Check sheet for the modelled part. Datum: model origin and axes. Units: mm. A direction names the side the tool comes from. Coordinates: 2 decimals unless noted, no trailing zeros. Loops run counter-clockwise (first coordinate to the right, second up) from the corner with the lowest first, then second, coordinate; pieces in that order, holes last. Notation, with made-up numbers: M -25.75,65 L -19.75,65 A22 ccw -19.75,88 Z; hole C -27,72 d3. An arc over 180 degrees is marked long. Answer as CSV lines item,"result". Start each with the question number.
from build123d import *

# Parameters (mm, degrees)
BOSS_EXTRUDE1_DEPTH = 5
BOSS_EXTRUDE2_DEPTH = 3
SKETCH3_W           = 7.507408842
SKETCH3_H           = 20
BOSS_EXTRUDE3_DEPTH = 12
SKETCH5_W           = 19.5
SKETCH5_H           = 2.15
CUT_EXTRUDE2_DEPTH  = 18
CUT_EXTRUDE3_DEPTH  = 50.600358979


with BuildPart() as part:
    # Sketch1 → Boss-Extrude1 (new body)
    with BuildSketch(Plane(origin=(0, 0, 0), x_dir=(1, 0, 0), z_dir=(0, 1, 0))):
        Polygon((10.024698463, 8.496116817), (-10.024698463, 8.496116817), (-29.349158436, -10.828343156), (-17.64879837, -38.142135624), (17.64879837, -38.142135624), (29.349158436, -10.828343156), align=None)
        Polygon((9.196271338, 6.496116817), (-9.196271338, 6.496116817), (-26.977652736, -11.28526458), (-16.329759674, -36.142135624), (16.329759674, -36.142135624), (26.977652736, -11.28526458), align=None, mode=Mode.SUBTRACT)
    extrude(amount=BOSS_EXTRUDE1_DEPTH)

    # Sketch2 → Boss-Extrude2 (add)
    with BuildSketch(Plane(origin=(0, 0, 0), x_dir=(-1, 0, 0), z_dir=(0, -1, 0))):
        Polygon((17.64879837, -38.142135624), (-17.64879837, -38.142135624), (-29.349158436, -10.828343156), (-10.024698463, 8.496116817), (10.024698463, 8.496116817), (29.349158436, -10.828343156), align=None)
    extrude(amount=BOSS_EXTRUDE2_DEPTH)

    # Sketch3 → Boss-Extrude3 (add)
    with BuildSketch(Plane(origin=(0, -3, 0), x_dir=(-1, 0, 0), z_dir=(0, -1, 0))):
        with Locations((9.003704421, -17.503883183)):
            Rectangle(SKETCH3_W, SKETCH3_H)
        with Locations((-9.003704421, -17.503883183)):
            Rectangle(SKETCH3_W, SKETCH3_H)
    extrude(amount=BOSS_EXTRUDE3_DEPTH)

    # Sketch5 → Cut-Extrude2 (cut)
    with BuildSketch(Plane(origin=(0, 0, 7.503883183), x_dir=(-1, 0, 0), z_dir=(0, 0, -1))):
        with Locations((0, -11.925)):
            Rectangle(SKETCH5_W, SKETCH5_H)
    extrude(amount=-CUT_EXTRUDE2_DEPTH, mode=Mode.SUBTRACT)

    # Sketch6 → Cut-Extrude3 (cut, through all)
    with BuildSketch(Plane(origin=(0, -3, 0), x_dir=(-1, 0, 0), z_dir=(0, -1, 0))):
        Polygon((5.25, -7.503883183), (5.25, -30.503883183), (-5.25, -30.503883183), (-5.25, -5.503883183), (-5.25, -3.503883183), (5.25, -3.503883183), align=None)
        Polygon((-24.606147036, -11.742186005), (-15.757408842, -32.399037357), (-15.757408842, -2.893447811), align=None)
        Polygon((-12.219190477, 0.676990597), (12.219190477, 0.676990597), (0, 4.412772028), align=None)
        Polygon((15.757408842, -2.893447811), (24.606147036, -11.742186005), (15.757408842, -32.399037357), align=None)
    extrude(amount=-CUT_EXTRUDE3_DEPTH, mode=Mode.SUBTRACT)


solid = part.part
Item 1: Sectioned sample at D-D, the plane z = -2. Record the boundary of the cut face in (x, y).
Item 2: Set-up check for faces 1 (the face through (15.757, -2, 18)), 2 (the face through (-7, -10.85, 16)), 3 (the face through (21.58, 2.46, 23.89)): record each of +Z, -Z, +X, -X, +Y, -Y from which the full face is reachable in a straight line by a thin tool's end or side.
Item 3: Go/stop test with flat-tipped pins: pin 1 (1.1 mm diameter, centred on x = -7.5, y = -12.5, fed in from -Z); pin 2 (12 mm diameter, centred on y = 1, z = 28, fed in from +X); pin 3 (12 mm diameter, centred on y = -11, z = 15, fed in from -X). Record where each tip stops, or that it passes through.
Item 4: Release check for a two-part mould opening along Z. For faces 4 (the face through (9, -9, 27.504)), 5 (the face through (9.75, -12, 16)), 6 (the face through (-6, 0, 15)) record: released by +Z, released by -Z, zero draft, split by the parting line, or undercut.
Item 5: Sectioned sample at B-B, the plane y = 3. Record the boundary of the cut face in (x, z).
Item 6: Sectioned sample at C-C, the plane x = 22.5. Record the boundary of the cut face in (y, z), and give its area (3 significant figures).
Item 7: Sectioned sample at A-A, the plane y = -7.25. Record the boundary of the cut face in (x, z), and give its area (3 significant figures).
Item 8: Material ranges on line 1 (Z direction, x = -5, y = 2); line 2 (X direction, y = -2.75, z = 9); line 3 (Y direction, x = 6.5, z = 13), recorded low to high. Write a range as from..to.
Reply:
1,outline,"M -16.52,-3 L -7.89,-3 L -7.89,0 L -13.69,0 L -13.69,5 L -16.52,5 Z; M 7.89,-3 L 16.52,-3 L 16.52,5 L 13.69,5 L 13.69,0 L 7.89,0 Z"
2,face 1,"+Y, -Y"
2,face 2,"-Z"
2,face 3,"+Y"
3,pin 1,"z = 7.5"
3,pin 2,"x = 24.56"
3,pin 3,"x = -12.76"
4,face 4,"released by +Z"
4,face 5,"zero draft"
4,face 6,"undercut"
5,outline,"M -29.35,10.83 L -10.02,-8.5 L 10.02,-8.5 L 29.35,10.83 L 17.65,38.14 L -17.65,38.14 Z; hole M -26.98,11.29 L -9.2,-6.5 L 9.2,-6.5 L 26.98,11.29 L 16.33,36.14 L -16.33,36.14 Z"
6,outline,"M -3,3.98 L 5,3.98 L 5,6.81 L 0,6.81 L 0,9.64 L -3,9.64 Z; M -3,16.66 L 0,16.66 L 0,21.74 L 5,21.74 L 5,26.82 L -3,26.82 Z"
6,area,"87.0 mm²"
7,outline,"M -12.76,7.5 L -5.25,7.5 L -5.25,27.5 L -12.76,27.5 Z; M 5.25,7.5 L 12.76,7.5 L 12.76,27.5 L 5.25,27.5 Z"
7,area,"300 mm²"
8,line 1,"-8.5..-6.5, 36.14..38.14"
8,line 2,"-27.52..-21.86, -15.76..-5.25, 5.25..15.76, 21.86..27.52"
8,line 3,"-15..-13, -10.85..0"
